from build123d import *

# Parameters (mm, degrees)
F0_W     = 3.5
F0_H     = 16
F1_DEPTH = 2
F2_D     = 3.15
F2_DEPTH = 15
F2_TIP   = 0.946355475


with BuildPart() as f1:
    # F0 (on Top) → F1 (new body)
    with BuildSketch(Plane.XY):
        Polygon((25, 26.0119763464), (-25, 26.0119763464), (-25, 6.0119763464), (-45, 6.0119763464), (-45, -15.4880236536), (-14.9, -15.4880236536), (-14.9, -6.9880236536), (-14.9, -3.9880236536), (4.5327088445, -3.9880236536), (4.5327088445, -6.9880236536), (14.9, -6.9880236536), (14.9, -15.4880236536), (45, -15.4880236536), (45, 6.0119763464), (25, 6.0119763464), align=None)
        with Locations((-16.65, 10.5119763464)):
            Rectangle(F0_W, F0_H, mode=Mode.SUBTRACT)
        with Locations((16.65, 10.5119763464)):
            Rectangle(F0_W, F0_H, mode=Mode.SUBTRACT)
    extrude(amount=F1_DEPTH)

    # F2
    with Locations(Plane(origin=(0, 0, 0), x_dir=(1, 0, 0), z_dir=(0, 0, -1))):
        with Locations((-42.1624206811, -0.5119763464), (-21.1624206811, -0.5119763464), (-21.1624206811, 12.9880236536), (-42.1624206811, 12.9880236536), (21.1624206811, 12.9880236536), (21.1624206811, -0.5119763464), (42.1624206811, -0.5119763464), (42.1624206811, 12.9880236536)):
            Hole(F2_D / 2, depth=F2_DEPTH)
            with Locations((0, 0, -(F2_DEPTH + F2_TIP / 2))):  # 118° drill point
                Cone(0, F2_D / 2, F2_TIP, mode=Mode.SUBTRACT)


solid = f1.part
Check sheet for the modelled part. Datum: model origin and axes. Units: mm. A direction names the side the tool comes from. Give positions to 0.01 mm unless a question says otherwise; leave off trailing zeros. Loops run counter-clockwise (first coordinate to the right, second up) from the corner with the lowest first, then second, coordinate; pieces in that order, holes last. Notation, with made-up numbers: M -33,62 L -11,62 A25 cw -11,74 Z; hole C -8,-21.75 d10. An arc over 180 degrees is marked long. Use a Markdown table: item, result. Add a question column.
Q1. Go/stop test with a flat-tipped pin: pin 1 (12 mm diameter, centred on x = 10.5, y = -1, fed in from -Z). Record where the tip stops, or that it passes through.
Q2. Mould release check, pull along X, two halves, no side actions. Record for faces 1 (the flat face through (-30, -15.488, 1)), 2 (the flat face through (-17, 2.512, 1)), 3 (the flat face through (25, 16, 1)): pulls with the +X half, pulls with the -X half, needs draft (parallel to the pull), parting line crosses it, or undercut.
Q3. Sectioned sample at A-A, the plane y = 7. Record the cut outline in (x, z), then the cut area to 3 significant figures.
Q4. Tool access check on faces 4 (the flat face through (30, -15.488, 1)), 5 (the flat face through (10, -6.988, 1)), 6 (the flat face through (18.4, 10, 1)). Record the directions out of +Z, -Z, +X, -X, +Y, -Y that give a thin tool (end or side, any length) a straight path to the whole face; none if there is none.
Q5. Sectioned sample at D-D, the plane y = 20. Record the cut outline in (x, z), then the cut area to 3 significant figures.
Q6. Scan lines: line 1 along X through (y, z) = (17.5, 1.05); line 2 along X through (y, z) = (0.5, 1.2); line 3 along X through (y, z) = (4.5, 1.9). Record each from-to range of solid material in increasing order. Write a range as [from, to].
Q7. Sectioned sample at C-C, the plane x = 5.5. Record the cut outline in (y, z), then the cut area to 3 significant figures.
Q8. Sectioned sample at B-B, the plane z = 0.95. Give the number of separate pieces and of enclosed holes in the cut face, then the cut area to 3 significant figures.
Verdict:
| question | item | result |
|---|---|---|
| 1 | pin 1 | z = 0 |
| 2 | face 1 | needs draft |
| 2 | face 2 | undercut |
| 2 | face 3 | pulls with the +X half |
| 3 | outline | M -25,0 L -18.4,0 L -18.4,2 L -25,2 Z; M -14.9,0 L 14.9,0 L 14.9,2 L -14.9,2 Z; M 18.4,0 L 25,0 L 25,2 L 18.4,2 Z |
| 3 | area | 86.0 mm^2 |
| 4 | face 4 | +Z, -Z, +X, -X, -Y |
| 4 | face 5 | +Z, -Z, -Y |
| 4 | face 6 | +Z, -Z |
| 5 | outline | M -25,0 L 25,0 L 25,2 L -25,2 Z |
| 5 | area | 100 mm^2 |
| 6 | line 1 | [-25, -18.4], [-14.9, 14.9], [18.4, 25] |
| 6 | line 2 | [-45, -43.74], [-40.59, -22.74], [-19.59, 19.59], [22.74, 40.59], [43.74, 45] |
| 6 | line 3 | [-45, -18.4], [-14.9, 14.9], [18.4, 45] |
| 7 | outline | M -6.99,0 L 26.01,0 L 26.01,2 L -6.99,2 Z |
| 7 | area | 66.0 mm^2 |
| 8 | separate pieces | 1 |
| 8 | enclosed holes | 10 |
| 8 | area | 2,450 mm^2 |
